Geometry: final body of the model. Coordinates: model frame, mm. Round coordinates to 2 decimals unless told otherwise and drop trailing zeros. Loops run counter-clockwise (first coordinate to the right, second up) from the corner with the lowest first, then second, coordinate; pieces in that order, holes last. Notation, with made-up numbers: M 64,26.5 L 122,26.5 A26 ccw 122,48.5 Z; hole C 83,9.25 d10. An arc over 180 degrees is marked long. Answer as a JSON object with one key per item and string values.
from build123d import *

# Parameters (mm, degrees)
ESBO_O1_R                = 1.6
RESSALTO_EXTRUS_O1_DEPTH = 6


with BuildPart() as part:
    # Esboço1 → Ressalto-extrusão1 (new body)
    with BuildSketch(Plane.XZ.offset(18)):
        with BuildLine():
            Line((-3.107348146, -5), (-1.107348146, -5))
            ThreePointArc((-1.107348146, -5), (3.892651854, 0), (-1.107348146, 5))
            Line((-1.107348146, 5), (-3.107348146, 5))
            ThreePointArc((-3.107348146, 5), (-8.107348146, 0), (-3.107348146, -5))
        make_face()
        Circle(ESBO_O1_R, mode=Mode.SUBTRACT)
    extrude(amount=-RESSALTO_EXTRUS_O1_DEPTH)


solid = part.part
1) Section query B-B (x = 0). Return the cut outline in (y, z).
Results:
{"outline": "M -18,-4.88 L -12,-4.88 L -12,-1.6 L -18,-1.6 Z; M -18,1.6 L -12,1.6 L -12,4.88 L -18,4.88 Z"}
2) Section query A-A (z = 0). Return the cut outline in (x, y).
Results:
{"outline": "M -8.11,-18 L -1.6,-18 L -1.6,-12 L -8.11,-12 Z; M 1.6,-18 L 3.89,-18 L 3.89,-12 L 1.6,-12 Z"}
3) Ray query, line 1 (Z direction, x = 0, y = -15.1); line 2 (X direction, y = -16.9, z = -0.25); line 3 (X direction, y = -13, z = 2). Return the intervals inside material, ascending.
Results:
{"line 1": "-4.88 to -1.6, 1.6 to 4.88", "line 2": "-8.1 to -1.58, 1.58 to 3.89", "line 3": "-7.69 to 3.48"}
4) Section query C-C (y = -15.5). Return the cut outline in (x, z), and give its area (3 significant figures).
Results:
{"outline": "M -3.11,-5 L -1.11,-5 A5 ccw -1.11,5 L -3.11,5 A5 ccw Z; hole C 0,0 d3.2", "area": "90.5 mm2"}
5) Section query D-D (x = 2.25). Return the cut outline in (y, z), and give its area (3 significant figures).
Results:
{"outline": "M -18,-3.71 L -12,-3.71 L -12,3.71 L -18,3.71 Z", "area": "44.5 mm2"}
6) Pull-direction query (Z, two-part tool) for faces 1 (the cylindrical face through (-8.106, -15.042, 0.11)), 2 (the cylindrical face through (-1.27, -15.04, -0.97)), 3 (the flat face through (-2, -12, 0)); classes: +Z half, -Z half, draft (parallel to the pull), parting line (faces both ways), or undercut.
Results:
{"face 1": "parting line", "face 2": "undercut", "face 3": "draft"}
